```python
from build123d import *

# Parameters (mm, degrees)
SKETCH_2_R          = 5
SKETCH_2_R_2        = 1.225
EXTRUDE_1_DEPTH     = 60
SKETCH_9_W          = 52
SKETCH_9_H          = 50
CUT_EXTRUDE_1_DEPTH = 60
SKETCH_10_R         = 1.225
CUT_EXTRUDE_2_DEPTH = 60


with BuildPart() as part:
    # 스케치2 → 보스-돌출1 (new body)
    with BuildSketch(Plane.XY):
        with BuildLine():
            Line((-14, 0), (-14, 40))
            Line((-14, 40), (14, 40))
            Line((14, 40), (14, 0))
            ThreePointArc((14, 0), (0, -14), (-14, 0))
        make_face()
        Circle(SKETCH_2_R, mode=Mode.SUBTRACT)
        with Locations((0, 11)):
            Circle(SKETCH_2_R_2, mode=Mode.SUBTRACT)
        with Locations((7.778174593, 7.778174593)):
            Circle(SKETCH_2_R_2, mode=Mode.SUBTRACT)
        with Locations((11, 0)):
            Circle(SKETCH_2_R_2, mode=Mode.SUBTRACT)
        with Locations((7.778174593, -7.778174593)):
            Circle(SKETCH_2_R_2, mode=Mode.SUBTRACT)
        with Locations((0, -11)):
            Circle(SKETCH_2_R_2, mode=Mode.SUBTRACT)
        with Locations((-7.778174593, -7.778174593)):
            Circle(SKETCH_2_R_2, mode=Mode.SUBTRACT)
        with Locations((-11, 0)):
            Circle(SKETCH_2_R_2, mode=Mode.SUBTRACT)
        with Locations((-7.778174593, 7.778174593)):
            Circle(SKETCH_2_R_2, mode=Mode.SUBTRACT)
    extrude(amount=EXTRUDE_1_DEPTH)

    # 스케치9 → 컷-돌출1 (cut)
    with BuildSketch(Plane(origin=(14, 0, 0), x_dir=(0, 0, -1), z_dir=(1, 0, 0))):
        with Locations((-30, 11)):
            Rectangle(SKETCH_9_W, SKETCH_9_H)
    extrude(amount=-CUT_EXTRUDE_1_DEPTH, mode=Mode.SUBTRACT)

    # 스케치10 → 컷-돌출2 (cut)
    with BuildSketch(Plane(origin=(0, 40, 0), x_dir=(1, 0, 0), z_dir=(0, 1, 0))):
        with Locations(Location((-7.774774878, -22.215482705, 0), (0, 0, 270))):
            Circle(SKETCH_10_R)
        with Locations(Location((0.003399715, -18.993657298, 0), (0, 0, 270))):
            Circle(SKETCH_10_R)
        with Locations(Location((7.781574308, -22.215482705, 0), (0, 0, 270))):
            Circle(SKETCH_10_R)
        with Locations(Location((11.003399715, -29.993657298, 0), (0, 0, 270))):
            Circle(SKETCH_10_R)
        with Locations(Location((7.781574308, -37.771831891, 0), (0, 0, 270))):
            Circle(SKETCH_10_R)
        with Locations(Location((0.003399715, -40.993657298, 0), (0, 0, 270))):
            Circle(SKETCH_10_R)
        with Locations(Location((-7.774774878, -37.771831891, 0), (0, 0, 270))):
            Circle(SKETCH_10_R)
        with Locations(Location((-10.996600285, -29.993657298, 0), (0, 0, 270))):
            Circle(SKETCH_10_R)
    extrude(amount=-CUT_EXTRUDE_2_DEPTH, mode=Mode.SUBTRACT)


solid = part.part
```
Build history of the part. All positions in model axes, mm. A direction names the side the tool comes from. Coordinates: 2 decimals unless noted, no trailing zeros. Order: outer loops, then holes, each group sorted by start corner. A loop starts at its lowest first (then second) coordinate and runs counter-clockwise, first axis right, second up.
Item 1: Drill centre lines: L1, parallel to X at y = 0, z = 59.1 (3 decimals); L2, parallel to Y at x = 0, z = 1.3 (3 decimals); L3, parallel to Z at x = -4, y = 22. Where is each one in solid material? Low to high.
Filled in:
L1: x = -14 to -12.225, -9.775 to -5, 5 to 9.775, 12.225 to 14
L2: y = -14 to -12.225, -9.775 to -5, 5 to 9.775, 12.225 to 40
L3: z = 0 to 4, 56 to 60
Item 2: Drop a flat-ended pin along its axis: pin 1 Ø3 at (x, z) = (6.5, 20.5) entering from -Y. Give the stop position or say it passes through.
Filled in:
pin 1: stops at y = 36
Item 3: Saw through at A-A on y = 16. List the corners of the cut face in (x, z).
Filled in:
outline: (-14, 0) - (14, 0) - (14, 4) - (-14, 4) - close; (-14, 56) - (14, 56) - (14, 60) - (-14, 60) - close
Item 4: Saw through at D-D on z = 7.5. List the corners of the cut face in (x, y), then the cut area to 3 significant figures.
Filled in:
outline: (-14, 36) - (14, 36) - (14, 40) - (-14, 40) - close
area: 112 mm2
Item 5: Mould opens along Y. For faces 3 (the flat face through (0, 36, 30)), 4 (the cylindrical face through (-12.224, 0.054, 57.972)), 5 (the cylindrical face through (-7.72, 38.03, 36.55)), 6 (the cylindrical face through (8.343, -8.865, 57.972)) say: released by +Y, released by -Y, zero draft, split by the parting line, or undercut.
Filled in:
face 3: released by -Y
face 4: undercut
face 5: zero draft
face 6: undercut
Item 6: Saw through at C-C on y = -11. List the corners of the cut face in (x, z) (3 decimals), then the cut area to 3 significant figures.
Filled in:
outline: (-8.66, 0) - (-1.225, 0) - (-1.225, 4) - (-8.66, 4) - close; (-8.66, 56) - (-1.225, 56) - (-1.225, 60) - (-8.66, 60) - close; (1.225, 0) - (8.66, 0) - (8.66, 4) - (1.225, 4) - close; (1.225, 56) - (8.66, 56) - (8.66, 60) - (1.225, 60) - close
area: 119 mm2
Item 7: Tool access for faces 1 (the flat face through (0, 16, 4)), 2 (the flat face through (0, 13, 60)): list every direction of +Z, -Z, +X, -X, +Y, -Y with a clear straight run to the whole face (end or side of a thin tool).
Filled in:
face 1: +X, -X, -Y
face 2: +Z, +X, -X, +Y, -Y
Item 8: Saw through at B-B on x = -3.75. List the corners of the cut face in (y, z), then the cut area to 3 significant figures.
Filled in:
outline: (-13.49, 0) - (-3.31, 0) - (-3.31, 4) - (-13.49, 4) - close; (-13.49, 56) - (-3.31, 56) - (-3.31, 60) - (-13.49, 60) - close; (3.31, 0) - (40, 0) - (40, 60) - (3.31, 60) - (3.31, 56) - (36, 56) - (36, 4) - (3.31, 4) - close
area: 583 mm2
